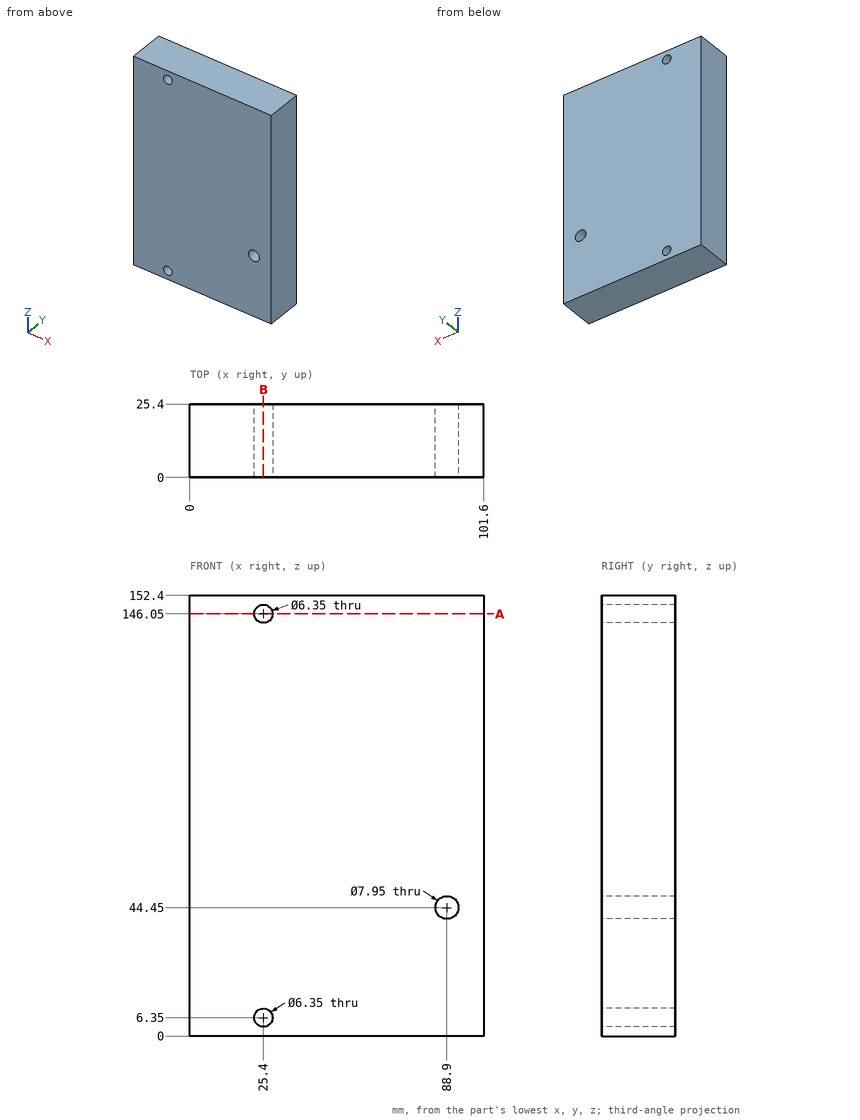
Input: dimensioned drawing with shaded views. Units: mm. Origin: part minimum x, y, z. Round coordinates to 2 decimals unless told otherwise and drop trailing zeros. Loops run counter-clockwise (first coordinate to the right, second up) from the corner with the lowest first, then second, coordinate; pieces in that order, holes last.
1) Section query B-B on x = 25.4. Return the cut outline in (y, z) (3 decimals), plus the area to 3 significant figures.
Ans:
outline: (0, 0) - (25.4, 0) - (25.4, 3.175) - (0, 3.175) - close; (0, 9.525) - (25.4, 9.525) - (25.4, 142.875) - (0, 142.875) - close; (0, 149.225) - (25.4, 149.225) - (25.4, 152.4) - (0, 152.4) - close
area: 3,550 mm2
2) Pin query (flat end, axial travel): pin 1 (4 mm diameter, centred on x = 25.4, z = 6.35, fed in from -Y). Return the tip coordinate at first contact, or that it passes through.
Ans:
pin 1: passes through
3) Section query A-A on z = 146.05. Return the cut outline in (x, y) (3 decimals).
Ans:
outline: (0, 0) - (22.225, 0) - (22.225, 25.4) - (0, 25.4) - close; (28.575, 0) - (101.6, 0) - (101.6, 25.4) - (28.575, 25.4) - close
4) Material intervals for line 1 (Z direction, x = 25.4, y = 5.5) (3 decimals); line 2 (Z direction, x = 88.9, y = 14.75) (1 decimal); line 3 (X direction, y = 16.25, z = 146.05) (3 decimals), sorted ascending.
Ans:
line 1: z = 0 to 3.175, 9.525 to 142.875, 149.225 to 152.4
line 2: z = 0 to 40.5, 48.4 to 152.4
line 3: x = 0 to 22.225, 28.575 to 101.6
